```python
from build123d import *

# Parameters (mm, degrees)
THICKEN2_START      = 118.58
THICKEN2_OUTLINE_W  = 5
THICKEN2_OUTLINE_H  = 308
THICKEN2_DEPTH      = 745
BOSS_EXTRUDE1_DEPTH = 10
SKETCH3_R           = 1.5
CUT_EXTRUDE1_DEPTH  = 298
FILLET1_R           = 5
FILLET2_R           = 5
BOSS_EXTRUDE2_DEPTH = 5
SKETCH5_R           = 98.944012136
SKETCH5_R_2         = 88.132026091
CUT_EXTRUDE2_DEPTH  = 2


# Read off the part's stored shape, not the designer's step: Thicken2
with BuildPart() as part:
    # Thicken2 outline → Thicken2 (new body)
    with BuildSketch(Plane.YZ.offset(THICKEN2_START)):
        with Locations((347.987717935, 154)):
            Rectangle(THICKEN2_OUTLINE_W, THICKEN2_OUTLINE_H)
    extrude(amount=THICKEN2_DEPTH)

    # Sketch2 → Boss-Extrude1 (add)
    with BuildSketch(Plane.XY.offset(308)):
        with BuildLine():
            Line((168.58, 350.487717935), (168.58, 360.487717935))
            ThreePointArc((168.58, 360.487717935), (178.58, 370.487717935), (188.58, 360.487717935))
            Line((188.58, 360.487717935), (188.58, 350.487717935))
            Line((188.58, 350.487717935), (168.58, 350.487717935))
        make_face()
        with BuildLine():
            Line((338.58, 350.487717935), (338.58, 360.487717935))
            ThreePointArc((338.58, 360.487717935), (348.58, 370.487717935), (358.58, 360.487717935))
            Line((358.58, 360.487717935), (358.58, 350.487717935))
            Line((358.58, 350.487717935), (338.58, 350.487717935))
        make_face()
        with BuildLine():
            Line((623.58, 350.487717935), (623.58, 360.487717935))
            ThreePointArc((623.58, 360.487717935), (633.58, 370.487717935), (643.58, 360.487717935))
            Line((643.58, 360.487717935), (643.58, 350.487717935))
            Line((643.58, 350.487717935), (623.58, 350.487717935))
        make_face()
        with BuildLine():
            Line((793.58, 350.487717935), (793.58, 360.487717935))
            ThreePointArc((793.58, 360.487717935), (803.58, 370.487717935), (813.58, 360.487717935))
            Line((813.58, 360.487717935), (813.58, 350.487717935))
            Line((813.58, 350.487717935), (793.58, 350.487717935))
        make_face()
    boss_extrude1 = extrude(amount=-BOSS_EXTRUDE1_DEPTH)

    # Sketch3 → Cut-Extrude1 (cut)
    with BuildSketch(Plane.XY.offset(308)):
        with Locations((178.58, 360.487717935)):
            Circle(SKETCH3_R)
        with Locations((348.58, 360.487717935)):
            Circle(SKETCH3_R)
        with Locations((633.58, 360.487717935)):
            Circle(SKETCH3_R)
        with Locations((803.58, 360.487717935)):
            Circle(SKETCH3_R)
    cut_extrude1 = extrude(amount=-CUT_EXTRUDE1_DEPTH, mode=Mode.SUBTRACT)

    # Fillet1
    fillet1_edges = [part.edges().sort_by_distance(p)[0] for p in [
        (188.58, 350.487717935, 303),
        (168.58, 350.487717935, 303),
        (358.58, 350.487717935, 303),
        (338.58, 350.487717935, 303),
        (643.58, 350.487717935, 303),
        (623.58, 350.487717935, 303),
        (813.58, 350.487717935, 303),
        (793.58, 350.487717935, 303),
    ]]
    fillet(fillet1_edges, radius=FILLET1_R)

    # Mirror2: Boss-Extrude1 across plane
    add(boss_extrude1.mirror(Plane.XY.offset(154)))

    # Mirror3: Cut-Extrude1 across plane
    add(cut_extrude1.mirror(Plane.XY.offset(154)), mode=Mode.SUBTRACT)

    # Fillet2
    fillet2_edges = [part.edges().sort_by_distance(p)[0] for p in [
        (168.58, 350.487717935, 5),
        (188.58, 350.487717935, 5),
        (338.58, 350.487717935, 5),
        (358.58, 350.487717935, 5),
        (623.58, 350.487717935, 5),
        (643.58, 350.487717935, 5),
        (793.58, 350.487717935, 5),
        (813.58, 350.487717935, 5),
    ]]
    fillet(fillet2_edges, radius=FILLET2_R)

    # Sketch4 → Boss-Extrude2 (add)
    with BuildSketch(Plane.XZ.offset(-345.487717935)):
        with BuildLine():
            Line((334.162131755, 308), (642.69967146, 308))
            ThreePointArc((642.69967146, 308), (706.409922047, 154), (642.69967146, 0))
            Line((642.69967146, 0), (334.162131755, 0))
            ThreePointArc((334.162131755, 0), (270.451881168, 154), (334.162131755, 308))
        make_face()
    extrude(amount=BOSS_EXTRUDE2_DEPTH)

    # Sketch5 → Cut-Extrude2 (cut)
    with BuildSketch(Plane.XZ.offset(-340.487717935)):
        with Locations(Location((482.249672024, 154, 0), (0, 0, 270))):
            Circle(SKETCH5_R)
        with Locations(Location((482.249672024, 154, 0), (0, 0, 270))):
            Circle(SKETCH5_R_2, mode=Mode.SUBTRACT)
    extrude(amount=-CUT_EXTRUDE2_DEPTH, mode=Mode.SUBTRACT)


solid = part.part
```
Can you work these out from the model? Positions are in its coordinate system, mm. A direction names the side the tool comes from. Coordinates: 2 decimals unless noted, no trailing zeros. Loops run counter-clockwise (first coordinate to the right, second up) from the corner with the lowest first, then second, coordinate; pieces in that order, holes last. Notation, with made-up numbers: (7.25, -11.75) -> (41.25, -11.75) arc R21 ccw to (41.25, -1.75) -> close; hole circle Ø5 at (-34.5, 15.5). An arc over 180 degrees is marked (long way). Put each result on its own line as item: value. Start each with the question number.
Q1. I want a section at A-A (z = 154). Write out the boundary of the cut face in (x, y).
Q2. If I drill on line 1 (Y direction, x = 633, z = 302); line 2 (X direction, y = 341.05, z = 154); line 3 (Y direction, x = 178.58, z = 305), over which ranges is the centre line in solid material (lowest first)? Write a range as [from, to].
Q3. I want a section at D-D (x = 548). Write out the boundary of the cut face in (y, z), plus the area to 3 significant figures.
Q4. I want a section at C-C (z = 21.5). Write out the boundary of the cut face in (x, y), plus the area to 3 significant figures.
Q5. I'm going to push flat-ended pins straight in: P1, Ø1.5, axis at y = 357, z = 303, coming from the +X side; P2, Ø2, axis at x = 754, z = 182.5, coming from the +Y side; P3, Ø5.5, axis at y = 357.5, z = 7, coming from the -X side. Where does each tip first touch, or does it pass through?
Q6. For faces 1 (the face through (706.397, 343.023, 156.394)), 2 (the face through (424.08, 342.488, 220.42)), 3 (the face through (270.465, 343.023, 151.606)), 4 (the face through (804, 358, 298)), which set-ups out of +Z, -Z, +X, -X, +Y, -Y let a thin tool reach every point of the face, with its end or its side?
Q7. I want a section at B-B (x = 261.5). Write out the boundary of the cut face in (y, z), plus the area to 3 significant figures.
Taken from the geometry:
1. outline: (118.58, 345.49) -> (270.45, 345.49) -> (270.45, 340.49) -> (383.31, 340.49) -> (383.31, 342.49) -> (394.12, 342.49) -> (394.12, 340.49) -> (570.38, 340.49) -> (570.38, 342.49) -> (581.19, 342.49) -> (581.19, 340.49) -> (706.41, 340.49) -> (706.41, 345.49) -> (863.58, 345.49) -> (863.58, 350.49) -> (118.58, 350.49) -> close
2. line 1: y = [340.49, 359.1], [361.87, 370.47]
2. line 2: x = [270.45, 383.31], [394.12, 570.38], [581.19, 706.41]
2. line 3: y = [345.49, 358.99], [361.99, 370.49]
3. outline: (340.49, 0) -> (350.49, 0) -> (350.49, 308) -> (340.49, 308) -> (340.49, 227.94) -> (342.49, 227.94) -> (342.49, 212.69) -> (340.49, 212.69) -> (340.49, 95.31) -> (342.49, 95.31) -> (342.49, 80.06) -> (340.49, 80.06) -> close
3. area: 3,020 mm2
4. outline: (118.58, 345.49) -> (315.35, 345.49) -> (315.35, 340.49) -> (661.52, 340.49) -> (661.52, 345.49) -> (863.58, 345.49) -> (863.58, 350.49) -> (118.58, 350.49) -> close
4. area: 5,460 mm2
5. P1: stops at x = 813.58
5. P2: stops at y = 350.49
5. P3: stops at x = 168.53
6. face 1: +X, -Y
6. face 2: -Y
6. face 3: -X, -Y
6. face 4: +X, -X, +Y
7. outline: (345.49, 0) -> (350.49, 0) -> (350.49, 308) -> (345.49, 308) -> close
7. area: 1,540 mm2
